```python
from build123d import *

# Parameters (mm, degrees)
SKETCH1_W           = 29.8
SKETCH1_H           = 22
SKETCH1_R           = 1
BOSS_EXTRUDE1_DEPTH = 2
SKETCH2_R           = 1
CUT_EXTRUDE1_DEPTH  = 10


with BuildPart() as part:
    # Sketch1 → Boss-Extrude1 (new body)
    with BuildSketch(Plane(origin=(0, 0, 0), x_dir=(1, 0, 0), z_dir=(0, 1, 0))):
        Rectangle(SKETCH1_W, SKETCH1_H)
        with Locations((10.15, 8)):
            Circle(SKETCH1_R, mode=Mode.SUBTRACT)
        with Locations((10.15, -8)):
            Circle(SKETCH1_R, mode=Mode.SUBTRACT)
        with Locations((-10.15, -8)):
            Circle(SKETCH1_R, mode=Mode.SUBTRACT)
        with Locations((-10.15, 8)):
            Circle(SKETCH1_R, mode=Mode.SUBTRACT)
    extrude(amount=BOSS_EXTRUDE1_DEPTH)

    # Sketch2 → Cut-Extrude1 (cut)
    with BuildSketch(Plane.XZ):
        with Locations((6.9, -5.25)):
            Circle(SKETCH2_R)
        with Locations((-6.9, -5.25)):
            Circle(SKETCH2_R)
    cut_extrude1 = extrude(amount=-CUT_EXTRUDE1_DEPTH, mode=Mode.SUBTRACT)

    # Mirror1: Cut-Extrude1 across plane
    add(cut_extrude1.mirror(Plane(origin=(0, 0, 0), x_dir=(1, 0, 0), z_dir=(0, 0, -1))), mode=Mode.SUBTRACT)


solid = part.part
```
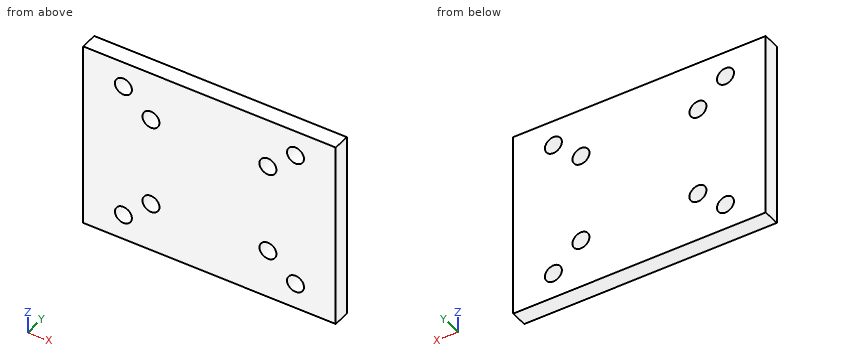
Build history of the part. All positions in model axes, mm. Coordinates: 2 decimals unless noted, no trailing zeros. Order: outer loops, then holes, each group sorted by start corner. A loop starts at its lowest first (then second) coordinate and runs counter-clockwise, first axis right, second up. Notation, with made-up numbers: M 0.25,34 L 38.25,34 A33 ccw 38.25,67 Z; hole C 78,-30 d11. An arc over 180 degrees is marked long. One line per question, with ' | ' between items. Start each with the question number.
1. Flat gauge pin, fed straight in: P1, Ø1.2, axis at x = 10.15, z = -8, coming from the +Y side. Where does the tip first touch, or does it go through?
2. Cut at C-C (y = 0.35). Count the separate pieces of the cut face and the enclosed holes in it, plus the area to 3 significant figures.
3. Cut at A-A (z = -8). Write the cut outline in (x, y), plus the area to 3 significant figures.
4. Cut at B-B (x = 10.15). Write the cut outline in (y, z), plus the area to 3 significant figures.
5. Wall check: line 1 along Z through (x, y) = (10.15, 1.35); line 2 along X through (y, z) = (0.8, 5.25); line 3 along Z through (x, y) = (6.9, 1.2). Give the ranges that are in metal, low to high. Write a range as [from, to].
The answers:
1) P1: passes through
2) separate pieces: 1 | enclosed holes: 8 | area: 630 mm2
3) outline: M -14.9,0 L -11.15,0 L -11.15,2 L -14.9,2 Z; M -9.15,0 L 9.15,0 L 9.15,2 L -9.15,2 Z; M 11.15,0 L 14.9,0 L 14.9,2 L 11.15,2 Z | area: 51.6 mm2
4) outline: M 0,-11 L 2,-11 L 2,-9 L 0,-9 Z; M 0,-7 L 2,-7 L 2,7 L 0,7 Z; M 0,9 L 2,9 L 2,11 L 0,11 Z | area: 36.0 mm2
5) line 1: z = [-11, -9], [-7, 7], [9, 11] | line 2: x = [-14.9, -7.9], [-5.9, 5.9], [7.9, 14.9] | line 3: z = [-11, -6.25], [-4.25, 4.25], [6.25, 11]
